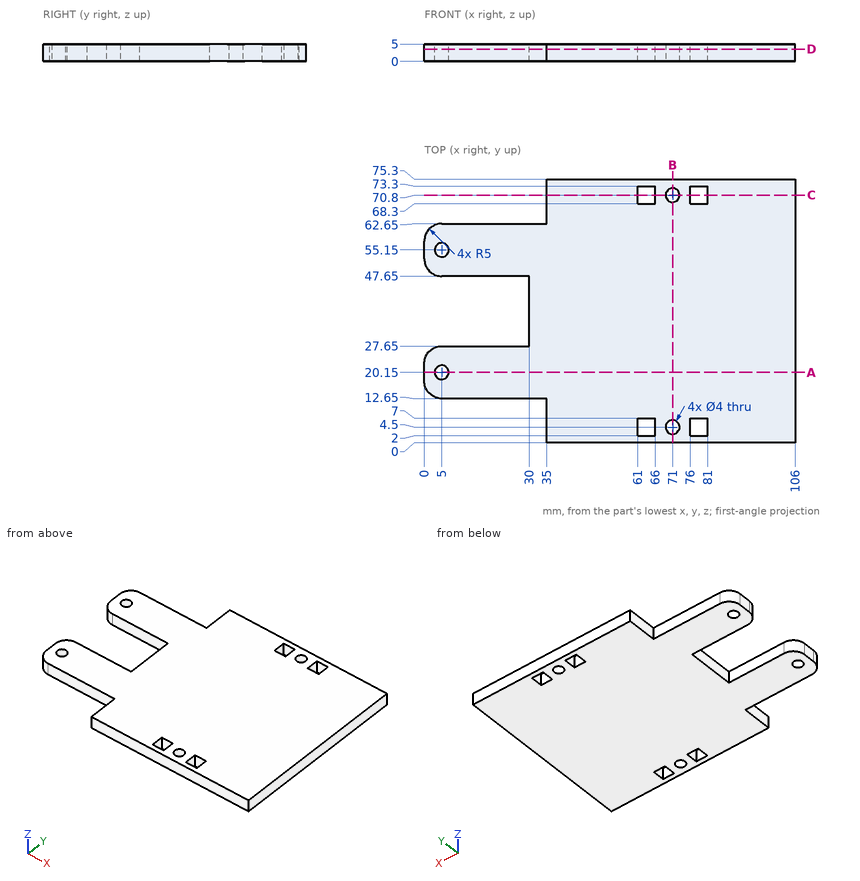
Could you check a few things on this drawing? It's one solid part, dimensions in mm from its lowest x, y, z. Coordinates: 2 decimals unless noted, no trailing zeros. Loops run counter-clockwise (first coordinate to the right, second up) from the corner with the lowest first, then second, coordinate; pieces in that order, holes last. Notation, with made-up numbers: (-39.75, -29) - (-4.75, -29) arc R12 cw to (-4.75, -15) - close; hole circle Ø6 at (33.5, 44.25). An arc over 180 degrees is marked (long way). Answer as a JSON object with one key per item and string values. Group by question number.
Item 1: If I drill on L1, parallel to Y at x = 80, z = 2.5; L2, parallel to Y at x = 71, z = 1.4; L3, parallel to Y at x = 5, z = 3.15, over which ranges is the centre line in solid material (lowest first)? Write a range as from..to.
Item 2: For pin 1 (1.5 mm diameter, centred on x = 21.5, z = 3, fed in from +Y); pin 2 (2.5 mm diameter, centred on y = 68.5, z = 2.5, fed in from -X); pin 3 (1.5 mm diameter, centred on x = 12.5, z = 2.5, fed in from -Y), each with a flat end and sliding along its axis, tell me the tip position at first contact or that it passes through.
Item 3: If we section it at C-C (y = 70.8): List the corners of the cut face in (x, z) for me.
Item 4: If we section it at D-D (z = 3.5): State how many separate pieces and enclosed holes the cut face has, plus the area to 3 significant figures.
Item 5: If we section it at B-B (x = 71): List the corners of the cut face in (y, z) for me.
Item 6: If we section it at A-A (y = 20.15): List the corners of the cut face in (x, z) for me.
Returned:
{
 "1": {"L1": "y = 0..2, 7..68.3, 73.3..75.3", "L2": "y = 0..2.5, 6.5..68.8, 72.8..75.3", "L3": "y = 12.65..18.15, 22.15..27.65, 47.65..53.15, 57.15..62.65"},
 "2": {"pin 1": "stops at y = 62.65", "pin 2": "stops at x = 35", "pin 3": "stops at y = 12.65"},
 "3": {"outline": "(35, 0) - (61, 0) - (61, 5) - (35, 5) - close; (66, 0) - (69, 0) - (69, 5) - (66, 5) - close; (73, 0) - (76, 0) - (76, 5) - (73, 5) - close; (81, 0) - (106, 0) - (106, 5) - (81, 5) - close"},
 "4": {"separate pieces": "1", "enclosed holes": "8", "area": "6,320 mm²"},
 "5": {"outline": "(0, 0) - (2.5, 0) - (2.5, 5) - (0, 5) - close; (6.5, 0) - (68.8, 0) - (68.8, 5) - (6.5, 5) - close; (72.8, 0) - (75.3, 0) - (75.3, 5) - (72.8, 5) - close"},
 "6": {"outline": "(0, 0) - (3, 0) - (3, 5) - (0, 5) - close; (7, 0) - (106, 0) - (106, 5) - (7, 5) - close"}
}
